from build123d import *

# Parameters (mm, degrees)
F0_W     = 285.75
F0_H     = 19.05
F1_DEPTH = 9.525
F0_R     = 28.575
F2_DEPTH = 12.7


with BuildPart() as f1:
    # F0 (on Top) → F1 (new body)
    with BuildSketch(Plane.XY):
        with Locations((114.3, -50.8)):
            Rectangle(F0_W, F0_H)
    extrude(amount=F1_DEPTH)

    # F0 (on Top) → F2 (join)
    with BuildSketch(Plane.XY):
        with BuildLine():
            Line((228.6, 76.2), (0, 76.2))
            ThreePointArc((0, 76.2), (-76.2, 0), (0, -76.2))
            Line((0, -76.2), (228.6, -76.2))
            ThreePointArc((228.6, -76.2), (304.8, 0), (228.6, 76.2))
        make_face()
        with Locations((114.3, -50.8)):
            Rectangle(F0_W, F0_H, mode=Mode.SUBTRACT)
        Circle(F0_R, mode=Mode.SUBTRACT)
        with Locations((76.2, 0)):
            Circle(F0_R, mode=Mode.SUBTRACT)
        with Locations((152.4, 0)):
            Circle(F0_R, mode=Mode.SUBTRACT)
        with Locations((228.6, 0)):
            Circle(F0_R, mode=Mode.SUBTRACT)
    extrude(amount=F2_DEPTH)


solid = f1.part
Source: CAD feature listing. Evaluate the final solid. Frame: model axes, mm. A direction names the side the tool comes from. Coordinates: 2 decimals unless noted, no trailing zeros. Order: outer loops, then holes, each group sorted by start corner. A loop starts at its lowest first (then second) coordinate and runs counter-clockwise, first axis right, second up.
Item 1: Cut plane C-C (z = 7.25). Return loops of the section in (x, y) (3 decimals), plus the area to 3 significant figures.
Output values:
outline: (0, -76.2) - (228.6, -76.2) arc R76.2 ccw to (228.6, 76.2) - (0, 76.2) arc R76.2 ccw to start; hole circle Ø57.15 at (0, 0); hole circle Ø57.15 at (76.2, 0); hole circle Ø57.15 at (152.4, 0); hole circle Ø57.15 at (228.6, 0)
area: 42,800 mm2
Item 2: Cut plane B-B (y = -8). Return loops of the section in (x, z), plus the area to 3 significant figures.
Output values:
outline: (-75.78, 0) - (-27.43, 0) - (-27.43, 12.7) - (-75.78, 12.7) - close; (27.43, 0) - (48.77, 0) - (48.77, 12.7) - (27.43, 12.7) - close; (103.63, 0) - (124.97, 0) - (124.97, 12.7) - (103.63, 12.7) - close; (179.83, 0) - (201.17, 0) - (201.17, 12.7) - (179.83, 12.7) - close; (256.03, 0) - (304.38, 0) - (304.38, 12.7) - (256.03, 12.7) - close
area: 2,040 mm2
Item 3: Pull-direction query (X, two-part tool) for faces 1 (the face through (-76.18, 1.68, 6.26)), 2 (the face through (112, 1, 0)), 3 (the face through (103.455, 8.583, 6.261)); classes: pulls with the +X half, pulls with the -X half, needs draft (parallel to the pull), parting line crosses it, or undercut.
Output values:
face 1: pulls with the -X half
face 2: needs draft
face 3: undercut
Item 4: First-contact query: P1, Ø1.6, axis at y = -53.5, z = 11.5, coming from the -X side; P2, Ø1, axis at y = -48, z = 10.5, coming from the +X side; P3, Ø1, axis at x = -17, z = 4, coming from the -Y side. Flat tips, straight axial feed; report the tip coordinate or a pass-through.
Output values:
P1: stops at x = -55.04
P2: stops at x = 288.18
P3: stops at y = -74.39
Item 5: Cut plane D-D (x = 151). Return loops of the section in (y, z) (3 decimals), plus the area to 3 significant figures.
Output values:
outline: (-76.2, 0) - (-28.541, 0) - (-28.541, 12.7) - (-41.275, 12.7) - (-41.275, 9.525) - (-60.325, 9.525) - (-60.325, 12.7) - (-76.2, 12.7) - close; (28.541, 0) - (76.2, 0) - (76.2, 12.7) - (28.541, 12.7) - close
area: 1,150 mm2
Item 6: Cut plane A-A (x = 76.2). Return loops of the section in (y, z) (3 decimals), plus the area to 3 significant figures.
Output values:
outline: (-76.2, 0) - (-28.575, 0) - (-28.575, 12.7) - (-41.275, 12.7) - (-41.275, 9.525) - (-60.325, 9.525) - (-60.325, 12.7) - (-76.2, 12.7) - close; (28.575, 0) - (76.2, 0) - (76.2, 12.7) - (28.575, 12.7) - close
area: 1,150 mm2
Item 7: Set-up query: faces 4 (the face through (116, 76.2, 6)), 5 (the face through (112, -51, 9.525)). Return all of +Z, -Z, +X, -X, +Y, -Y with unobstructed straight access to the full face (end or side cutting, diameter ignored); none if empty.
Output values:
face 4: +Z, -Z, +X, -X, +Y
face 5: +Z
Item 8: Material intervals for line 1 (Y direction, x = 76.2, z = 5.5) (3 decimals); line 2 (Z direction, x = 122.5, y = -50) (3 decimals); line 3 (Y direction, x = 64.5, z = 5), sorted ascending.
Output values:
line 1: y = -76.2 to -28.575, 28.575 to 76.2
line 2: z = 0 to 9.525
line 3: y = -76.2 to -26.07, 26.07 to 76.2
